from build123d import *

# Parameters (mm, degrees)
SKETCH1_R      = 2.794
EXTRUDE1_DEPTH = 51.816
SKETCH2_R      = 6.604
EXTRUDE2_DEPTH = 12.7
EXTRUDE3_START = -12.7
EXTRUDE3_DEPTH = 12.7
FILLET1_R      = 2.54
FILLET2_R      = 2.54


with BuildPart() as part:
    # Sketch1 → Extrude1 (new body)
    with BuildSketch(Plane.XY):
        Circle(SKETCH1_R)
    extrude(amount=EXTRUDE1_DEPTH)

    # Sketch2 → Extrude2 (add)
    with BuildSketch(Plane.XY.offset(51.816)):
        Circle(SKETCH2_R)
    extrude(amount=EXTRUDE2_DEPTH)

    # Sketch3 → Extrude3 (add)
    with BuildSketch(Plane.XY.offset(64.516).offset(EXTRUDE3_START)):
        with BuildLine():
            Line((-2.54, 15.122583735), (2.54, 15.122583735))
            ThreePointArc((2.54, 15.122583735), (3.016066659, 10.467431069), (3.175, 5.790698663))
            ThreePointArc((3.175, 5.790698663), (0, 6.604), (-3.175, 5.790698663))
            ThreePointArc((-3.175, 5.790698663), (-3.016066659, 10.467431069), (-2.54, 15.122583735))
        make_face()
        with BuildLine():
            Line((2.54, -15.122583735), (-2.54, -15.122583735))
            ThreePointArc((-2.54, -15.122583735), (-3.016066659, -10.467431069), (-3.175, -5.790698663))
            ThreePointArc((-3.175, -5.790698663), (0, -6.604), (3.175, -5.790698663))
            ThreePointArc((3.175, -5.790698663), (3.016066659, -10.467431069), (2.54, -15.122583735))
        make_face()
    extrude(amount=EXTRUDE3_DEPTH)

    # Fillet1
    fillet1_edges = [part.edges().sort_by_distance(p)[0] for p in [
        (-2.54, 15.122583735, 58.166),
        (2.54, 15.122583735, 58.166),
        (2.54, -15.122583735, 58.166),
        (-2.54, -15.122583735, 58.166),
    ]]
    fillet(fillet1_edges, radius=FILLET1_R)

    # Fillet2
    fillet2_edges = [part.edges().sort_by_distance(p)[0] for p in [
        (-3.175, 5.790698663, 58.166),
        (3.175, 5.790698663, 58.166),
        (3.175, -5.790698663, 58.166),
    ]]
    fillet(fillet2_edges, radius=FILLET2_R)
    fillet2_2_edges = [part.edges().sort_by_distance(p)[0] for p in [
        (-6.57965204, -0.566564238, 51.816),
        (3.047804414, 9.974982228, 64.516),
        (-3.047804414, 9.974982228, 51.816),
        (6.604, 0, 64.516),
        (6.604, 0, 51.816),
        (-3.084466617, -9.321288711, 64.516),
        (3.047804414, -9.974982228, 51.816),
        (-3.084466617, -9.321288711, 51.816),
        (0, -15.122583735, 64.516),
        (3.047804414, -9.974982228, 64.516),
        (0, 15.122583735, 64.516),
        (-3.047804414, 9.974982228, 64.516),
        (1.98808874, 14.468324748, 64.516),
        (-1.98808874, 14.468324748, 64.516),
        (1.98808874, -14.468324748, 64.516),
        (-1.98808874, -14.468324748, 64.516),
        (0, -15.122583735, 51.816),
        (0, 15.122583735, 51.816),
        (3.047804414, 9.974982228, 51.816),
        (1.98808874, 14.468324748, 51.816),
        (-1.98808874, 14.468324748, 51.816),
        (1.98808874, -14.468324748, 51.816),
        (-1.98808874, -14.468324748, 51.816),
        (-6.57965204, -0.566564238, 64.516),
        (-3.424141618, 6.02472451, 64.516),
        (3.424141618, 6.02472451, 51.816),
        (3.424141618, -6.02472451, 64.516),
        (3.424141618, -6.02472451, 51.816),
        (3.424141618, 6.02472451, 64.516),
        (-3.424141618, 6.02472451, 51.816),
    ]]
    fillet(fillet2_2_edges, radius=FILLET2_R)


solid = part.part
Input: part model. Units: mm. Frame: model coordinates. A direction names the side the tool comes from. Give positions to 0.01 mm unless a question says otherwise; leave off trailing zeros. Loops run counter-clockwise (first coordinate to the right, second up) from the corner with the lowest first, then second, coordinate; pieces in that order, holes last. Notation, with made-up numbers: M -32.5,35 L 7.5,35 A26 ccw 7.5,71 Z; hole C 2,-29.75 d7. An arc over 180 degrees is marked long. Use one line per item in the form item = value.
1. Line query: L1, parallel to Z at x = 1, y = 6; L2, parallel to X at y = -12.5, z = 54; L3, parallel to Y at x = -0.75, z = 40.5. Output: solid intervals per line, ascending.
Numbers:
L1 = 51.83 to 64.5
L2 = -2.82 to 2.82
L3 = -2.69 to 2.69
2. Section query A-A, the plane y = 0. Return the cut outline in (x, z).
Numbers:
outline = M -6.6,54.36 A2.54 ccw -4.06,51.82 L -2.79,51.82 L -2.79,0 L 2.79,0 L 2.79,51.82 L 4.06,51.82 A2.54 ccw 6.6,54.36 L 6.6,61.98 A2.54 ccw 4.06,64.52 L -4.06,64.52 A2.54 ccw -6.6,61.98 Z
3. Section query B-B, the plane z = 17.5. Return the cut outline in (x, y).
Numbers:
outline = C 0,0 d5.59
4. First-contact query: pin 1 (4 mm diameter, centred on x = 4, y = -7.5, fed in from -Z); pin 2 (2 mm diameter, centred on x = 5, z = 13.5, fed in from +Y); pin 3 (2 mm diameter, centred on y = 0, z = 17.5, fed in from +X); pin 4 (1.5 mm diameter, centred on x = -3, y = -5, fed in from +Z). Flat tips, straight axial feed; report the tip coordinate or a pass-through.
Numbers:
pin_1 = 52.23
pin_2 = through
pin_3 = 2.79
pin_4 = 64.3
5. Reachability of faces 1 (the face through (-3.08, -9.37, 58.11)), 2 (the face through (-2.217, -1.7, 25.545)) from +Z, -Z, +X, -X, +Y, -Y: full face, straight path, thin tool, end or side. Return the list, or none.
Numbers:
face_1 = +Z, -Z, -X, -Y
face_2 = -Z
